from build123d import *

# Parameters (mm, degrees)
SKETCH1_W           = 146.6
SKETCH1_H           = 70.6
BOSS_EXTRUDE1_DEPTH = 8.25
FILLET1_R           = 14
SKETCH2_R           = 7.8441354
SKETCH2_R_2         = 8.049819652
SKETCH2_R_3         = 8.178113635
BOSS_EXTRUDE2_DEPTH = 2


with BuildPart() as part:
    # Sketch1 → Boss-Extrude1 (new body)
    with BuildSketch(Plane(origin=(0, 0, 0), x_dir=(1, 0, 0), z_dir=(0, 1, 0))):
        Rectangle(SKETCH1_W, SKETCH1_H)
    extrude(amount=BOSS_EXTRUDE1_DEPTH)

    # Fillet1
    fillet1_edges = [part.edges().sort_by_distance(p)[0] for p in [
        (-73.3, 4.125, -35.3),
        (73.3, 4.125, -35.3),
        (73.3, 4.125, 35.3),
        (-73.3, 4.125, 35.3),
    ]]
    fillet(fillet1_edges, radius=FILLET1_R)

    # Sketch2 → Boss-Extrude2 (add)
    with BuildSketch(Plane(origin=(0, 8.25, 0), x_dir=(1, 0, 0), z_dir=(0, 1, 0))):
        with Locations(Location((39.929810702, 21.760044193, 0), (0, 0, 270))):
            Circle(SKETCH2_R)
        with Locations(Location((59.990850443, 22.050286799, 0), (0, 0, 270))):
            Circle(SKETCH2_R_2)
        with Locations(Location((50.210763803, 3.237335299, 0), (0, 0, 270))):
            Circle(SKETCH2_R_3)
    extrude(amount=BOSS_EXTRUDE2_DEPTH)


solid = part.part
Here's how the part is built. I have some questions about the finished solid (model axes, mm). Round coordinates to 2 decimals unless told otherwise and drop trailing zeros. Loops run counter-clockwise (first coordinate to the right, second up) from the corner with the lowest first, then second, coordinate; pieces in that order, holes last.
1. If we section it at D-D on z = -2: Write out the boundary of the cut face in (x, y).
Answer list:
outline: (-73.3, 0) - (73.3, 0) - (73.3, 8.25) - (58.29, 8.25) - (58.29, 10.25) - (42.13, 10.25) - (42.13, 8.25) - (-73.3, 8.25) - close
2. If we section it at A-A on y = 5: Write out the boundary of the cut face in (x, z).
Answer list:
outline: (-73.3, -21.3) arc R14 ccw to (-59.3, -35.3) - (59.3, -35.3) arc R14 ccw to (73.3, -21.3) - (73.3, 21.3) arc R14 ccw to (59.3, 35.3) - (-59.3, 35.3) arc R14 ccw to (-73.3, 21.3) - close
3. If we section it at C-C on x = -56.5: Write out the boundary of the cut face in (y, z), plus the area to 3 significant figures.
Answer list:
outline: (0, -35.3) - (8.25, -35.3) - (8.25, 35.3) - (0, 35.3) - close
area: 582 mm2
4. If we section it at B-B on z = -18.5: Write out the boundary of the cut face in (x, y).
Answer list:
outline: (-73.3, 0) - (73.3, 0) - (73.3, 8.25) - (67.22, 8.25) - (67.22, 10.25) - (52.77, 10.25) - (52.77, 8.25) - (47.06, 8.25) - (47.06, 10.25) - (32.8, 10.25) - (32.8, 8.25) - (-73.3, 8.25) - close
5. If I drill on line 1 along Y through (x, z) = (12, -2); line 2 along Z through (x, y) = (-64.5, 1.5); line 3 along X through (y, z) = (9, -10), over which ranges is the centre line in solid material (lowest first)?
Answer list:
line 1: y = 0 to 8.25
line 2: z = -34.3 to 34.3
line 3: x = 45.61 to 54.81
6. For P1, Ø2, axis at y = 7.5, z = -25, coming from the +X side, with a flat end and sliding along its axis, tell me the tip position at first contact or that it passes through.
Answer list:
P1: stops at x = 73.04
7. We'd pull the mould along X, two halves only. Please class faces 1 (the face through (42.227, 9.236, -5.01)), 2 (the face through (47.707, 9.236, -22.781)), 3 (the face through (67.97, 9.24, -23.1)), 4 (the face through (50, 10.25, -3)): +X half, -X half, draft (parallel to the pull), parting line (faces both ways), or undercut.
Answer list:
face 1: parting line
face 2: undercut
face 3: undercut
face 4: draft
